Read the model definition and answer for the solid it produces. Units are mm, in the model's axes. A direction names the side the tool comes from. Coordinates: 2 decimals unless noted, no trailing zeros. Write each loop counter-clockwise with the first axis right and the second up, starting at its lowest first coordinate (ties: lowest second). Pieces come first, ordered by that corner, then holes.
Item 1: Section C-C (z = -41) is taken. Give the vertices of the cut face in (x, y), then the cut area to 3 significant figures.
Item 2: Determine the mould class of faces 1 (the face through (-4.25, 5, -277)), 2 (the face through (-9, -15, 0)), 3 (the face through (-0.06, -2.87, -276.93)), 4 (the face through (0, 0, -290)) for opening direction Z: released by +Z, released by -Z, zero draft, split by the parting line, or undercut.
Item 3: Straight lines are drawn through the part: probe 1 along Y at (x, z) = (0, -270); probe 2 along Z at (x, y) = (15, 12); probe 3 along Y at (x, z) = (-4, -82). For each, find the intervals that lie inside material, in ascending order.
Item 4: Section A-A (y = 0) is taken. Give the vertices of the cut face in (x, z).
Item 5: Each of these flat-tipped pins is pushed along its axis until it touches: P1, Ø8, axis at x = -11, y = 9, coming from the -Z side; P2, Ø2, axis at y = 4.5, z = -192.5, coming from the -X side; P3, Ø2, axis at x = 6, z = -2, coming from the +Y side; P4, Ø12, axis at y = 0, z = -270, coming from the -X side. Where does it stop, or does it pass through?
Item 6: Section B-B (z = 29.5) is taken. Give the vertices of the cut face in (x, y).
Item 7: A tool of negligible diameter and unlimited length cuts with its end or side. For faces 5 (the face through (9.139, 14.334, 24.65)), 6 (the face through (13, 0, -250)), 7 (the face through (-2.6, -19.83, -135.21)), 8 (the face through (-14, 0, -250)), 9 (the face through (0, 0, 50)), from which of +Z, -Z, +X, -X, +Y, -Y can it reach the whole face along a straight path? Write none if from no direction.
from build123d import *

# Parameters (mm, degrees)
SKETCH5_R               = 20
BOSS_EXTRUDE4_DEPTH     = 250
SKETCH6_R               = 17
BOSS_EXTRUDE5_DEPTH     = 50
SKETCH7_R               = 7.5
BOSS_EXTRUDE6_DEPTH     = 4.25
CUT_EXTRUDE1_DEPTH      = 302.330383466
CUT_EXTRUDE1_DEPTH_BACK = 302.330383466
SKETCH8_OUTSIDE_W       = 110.934
SKETCH8_OUTSIDE_H       = 110.934
SKETCH8_OUTSIDE_R       = 20
FILLET1_R               = 5


with BuildPart() as part:
    # Sketch5 → Boss-Extrude4 (new body)
    with BuildSketch(Plane.XY):
        Circle(SKETCH5_R)
    extrude(amount=-BOSS_EXTRUDE4_DEPTH)

    # Sketch6 → Boss-Extrude5 (add)
    with BuildSketch(Plane.XY):
        Circle(SKETCH6_R)
    extrude(amount=BOSS_EXTRUDE5_DEPTH)

    # Sketch7 → Boss-Extrude6 (add, symmetric)
    with BuildSketch(Plane(origin=(0, 0, 0), x_dir=(0, 0, -1), z_dir=(1, 0, 0))):
        with BuildLine():
            Line((250, 20), (270, 20))
            ThreePointArc((270, 20), (290, 0), (270, -20))
            Line((270, -20), (250, -20))
            Line((250, -20), (250, 20))
        make_face()
        with Locations((270, 0)):
            Circle(SKETCH7_R, mode=Mode.SUBTRACT)
    extrude(amount=BOSS_EXTRUDE6_DEPTH, both=True)

    # Sketch8 outside → Cut-Extrude1 (cut, two sides: drawn at the far end of the back side and taken through both)
    with BuildSketch(Plane(origin=(0, 0, -250), x_dir=(-1, 0, 0), z_dir=(0, 0, -1)).offset(-CUT_EXTRUDE1_DEPTH_BACK)):
        Rectangle(SKETCH8_OUTSIDE_W, SKETCH8_OUTSIDE_H)
        with Locations(Location((0, 0, 0), (0, 0, 180))):
            Circle(SKETCH8_OUTSIDE_R, mode=Mode.SUBTRACT)
    extrude(amount=CUT_EXTRUDE1_DEPTH + CUT_EXTRUDE1_DEPTH_BACK, mode=Mode.SUBTRACT)

    # Fillet1
    fillet1_edges = [part.edges().sort_by_distance(p)[0] for p in [
        (4.25, 0, -250),
        (-4.25, 0, -250),
    ]]
    fillet(fillet1_edges, radius=FILLET1_R)


solid = part.part
Established:
1. outline: circle Ø40 at (0, 0)
1. area: 1,260 mm2
2. face 1: zero draft
2. face 2: released by +Z
2. face 3: undercut
2. face 4: released by -Z
3. probe 1: y = -20 to -7.5, 7.5 to 20
3. probe 2: z = -250 to 0
3. probe 3: y = -19.6 to 19.6
4. outline: (-20, -250) - (-9.25, -250) arc R5 cw to (-4.25, -255) - (-4.25, -262.5) - (4.25, -262.5) - (4.25, -255) arc R5 cw to (9.25, -250) - (20, -250) - (20, 0) - (17, 0) - (17, 50) - (-17, 50) - (-17, 0) - (-20, 0) - close; (-4.25, -290) - (4.25, -290) - (4.25, -277.5) - (-4.25, -277.5) - close
5. P1: stops at z = -250.53
5. P2: stops at x = -19.69
5. P3: stops at y = 19.36
5. P4: passes through
6. outline: circle Ø34 at (0, 0)
7. face 5: +Z
7. face 6: -Z, +X, +Y, -Y
7. face 7: +Z, -Z
7. face 8: -Z, -X, +Y, -Y
7. face 9: +Z, +X, -X, +Y, -Y
